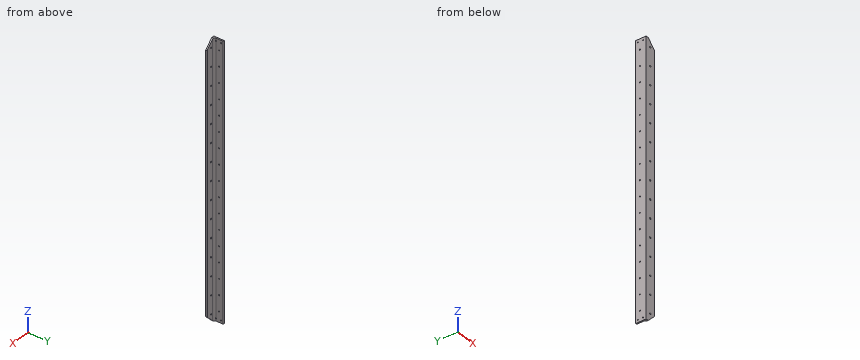
from build123d import *

# Parameters (mm, degrees)
AUFSATZ_LINEAR_AUSTRAGEN1_DEPTH      = 1040
SCHNITT_LINEAR_AUSTRAGEN1_DEPTH      = 10
SCHNITT_LINEAR_AUSTRAGEN1_DEPTH_BACK = 10
SKIZZE3_R                            = 3
SCHNITT_LINEAR_AUSTRAGEN2_DEPTH      = 10
LINEARES_MUSTER1_COUNT               = 15
LINEARES_MUSTER1_PITCH               = 70
LINEARES_MUSTER2_COUNT               = 17
LINEARES_MUSTER2_PITCH               = 60
M5_GEWINDEBOHRUNG2_D                 = 4.2
M5_GEWINDEBOHRUNG2_DEPTH             = 14
M5_GEWINDEBOHRUNG2_TIP               = 1.2618073


with BuildPart() as part:
    # Skizze1 → Aufsatz-Linear austragen1 (new body)
    with BuildSketch(Plane.XY):
        with BuildLine():
            Line((0, 40), (0, 0))
            Line((0, 0), (40, 0))
            Line((40, 0), (40, 1.5))
            ThreePointArc((40, 1.5), (38.974873734, 3.974873734), (36.5, 5))
            Line((36.5, 5), (12, 5))
            ThreePointArc((12, 5), (7.050252532, 7.050252532), (5, 12))
            Line((5, 12), (5, 36.5))
            ThreePointArc((5, 36.5), (3.974873734, 38.974873734), (1.5, 40))
            Line((1.5, 40), (0, 40))
        make_face()
    extrude(amount=AUFSATZ_LINEAR_AUSTRAGEN1_DEPTH)

    # Skizze2 → Schnitt-Linear austragen1 (cut, two sides: drawn at the far end of the back side and taken through both)
    with BuildSketch(Plane(origin=(0, 5, 0), x_dir=(1, 0, 0), z_dir=(0, 1, 0)).offset(-SCHNITT_LINEAR_AUSTRAGEN1_DEPTH_BACK)):
        Polygon((10, -1040), (40, -1010), (40, -1040), align=None)
        Polygon((10, 0), (40, -30), (40, 0), align=None)
    extrude(amount=SCHNITT_LINEAR_AUSTRAGEN1_DEPTH + SCHNITT_LINEAR_AUSTRAGEN1_DEPTH_BACK, mode=Mode.SUBTRACT)

    # Skizze3 → Schnitt-Linear austragen2 (cut)
    with BuildSketch(Plane(origin=(0, 5, 0), x_dir=(1, 0, 0), z_dir=(0, 1, 0))):
        with Locations(Location((20, -30, 0), (0, 0, 180))):
            Circle(SKIZZE3_R)
    schnitt_linear_austragen2 = extrude(amount=-SCHNITT_LINEAR_AUSTRAGEN2_DEPTH, mode=Mode.SUBTRACT)

    # Lineares Muster1: Schnitt-Linear austragen2 ×15
    with Locations(*[(0, 0, i * LINEARES_MUSTER1_PITCH) for i in range(1, LINEARES_MUSTER1_COUNT)]):
        add(schnitt_linear_austragen2, mode=Mode.SUBTRACT)

    # Skizze5 → M5 Gewindebohrung1 (revolve, cut)
    with BuildSketch(Plane(origin=(0, 24, 1000), x_dir=(0, 0, 1), z_dir=(0, 1, 0))):
        Polygon((0, 0), (0, 15.2618073), (2.1, 14), (2.1, 0), align=None)
    m5_gewindebohrung1 = revolve(axis=Axis((-6.35, 24, 1000), (1, 0, 0)), mode=Mode.SUBTRACT)

    # Lineares Muster2: M5 Gewindebohrung1 ×17
    with Locations(*[(0, 0, -i * LINEARES_MUSTER2_PITCH) for i in range(1, LINEARES_MUSTER2_COUNT)]):
        add(m5_gewindebohrung1, mode=Mode.SUBTRACT)

    # M5 Gewindebohrung2
    with Locations(Plane.ZY):
        with Locations((10, 32), (1030, 12), (1030, 32), (10, 12)):
            Hole(M5_GEWINDEBOHRUNG2_D / 2, depth=M5_GEWINDEBOHRUNG2_DEPTH)
            with Locations((0, 0, -(M5_GEWINDEBOHRUNG2_DEPTH + M5_GEWINDEBOHRUNG2_TIP / 2))):  # 118° drill point
                Cone(0, M5_GEWINDEBOHRUNG2_D / 2, M5_GEWINDEBOHRUNG2_TIP, mode=Mode.SUBTRACT)


solid = part.part
Can you work these out from the model? Positions are in its coordinate system, mm. Round coordinates to 2 decimals unless told otherwise and drop trailing zeros. Write each loop counter-clockwise with the first axis right and the second up, starting at its lowest first coordinate (ties: lowest second). Pieces come first, ordered by that corner, then holes. Notation, with made-up numbers: (-9.75, 19) -> (46.25, 19) arc R29 ccw to (46.25, 40) -> close; hole circle Ø8 at (-28, -22). An arc over 180 degrees is marked (long way). Use one line per item in the form item = value. Start each with the question number.
Q1. If I drill on probe 1 along X at (y, z) = (2.1, 170); probe 2 along X at (y, z) = (1.3, 1010); probe 3 along Y at (x, z) = (29.5, 534), over which ranges is the centre line in solid material (lowest first)? Write a range as [from, to].
Q2. I'm going to push flat-ended pins straight in: P1, Ø5, axis at y = 24, z = 880, coming from the +X side; P2, Ø5.5, axis at y = 12, z = 1030, coming from the +X side; P3, Ø9.5, axis at x = 20, z = 590, coming from the +Y side. Where does each tip first touch, or does it pass through?
Q3. Imagine slicing it at A-A (z = 297.5). Please give me the cut outline in (x, y).
Worked out:
q1.probe_1 = [0, 17], [23, 39.95]
q1.probe_2 = [0, 17], [23, 40]
q1.probe_3 = [0, 5]
q2.P1 = 5
q2.P2 = 5.56
q2.P3 = 5
q3.outline = (0, 0) -> (40, 0) -> (40, 1.5) arc R3.5 ccw to (36.5, 5) -> (12, 5) arc R7 cw to (5, 12) -> (5, 36.5) arc R3.5 ccw to (1.5, 40) -> (0, 40) -> close
